```python
from build123d import *

# Parameters (mm, degrees)
SKETCH_W  = 65
SKETCH_H  = 56
SKETCH_R  = 1.35
PAD_DEPTH = 2.5
FILLET_R  = 2


with BuildPart() as part:
    # Sketch → Pad (new body)
    with BuildSketch(Plane.XY):
        Rectangle(SKETCH_W, SKETCH_H)
        with Locations((15, 15)):
            Circle(SKETCH_R, mode=Mode.SUBTRACT)
        with Locations((15, -15)):
            Circle(SKETCH_R, mode=Mode.SUBTRACT)
        with Locations((-15, -15)):
            Circle(SKETCH_R, mode=Mode.SUBTRACT)
        with Locations((-15, 15)):
            Circle(SKETCH_R, mode=Mode.SUBTRACT)
        with Locations((-29, 24.5)):
            Circle(SKETCH_R, mode=Mode.SUBTRACT)
        with Locations((29, 24.5)):
            Circle(SKETCH_R, mode=Mode.SUBTRACT)
        with Locations((29, -24.5)):
            Circle(SKETCH_R, mode=Mode.SUBTRACT)
        with Locations((-29, -24.5)):
            Circle(SKETCH_R, mode=Mode.SUBTRACT)
    extrude(amount=PAD_DEPTH)

    # Fillet
    fillet_edges = [part.edges().sort_by_distance(p)[0] for p in [
        (-32.5, -28, 1.25),
        (-32.5, 28, 1.25),
        (32.5, -28, 1.25),
        (32.5, 28, 1.25),
    ]]
    fillet(fillet_edges, radius=FILLET_R)


solid = part.part
```
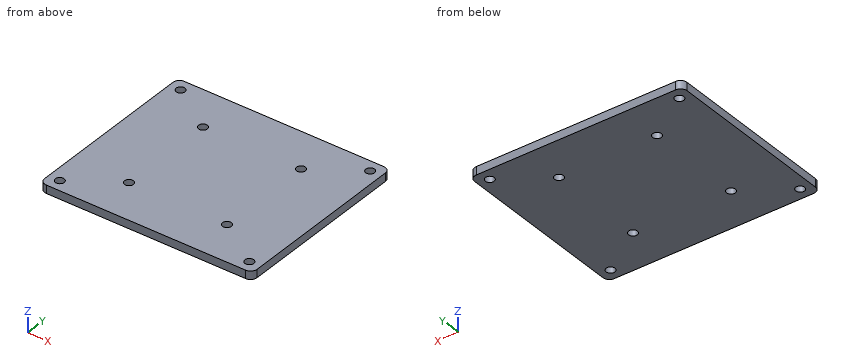
Verification items for the finished model (mm, model axes). Round coordinates to 2 decimals unless told otherwise and drop trailing zeros. Order: outer loops, then holes, each group sorted by start corner. A loop starts at its lowest first (then second) coordinate and runs counter-clockwise, first axis right, second up.
1) Cross-section at B-B, the plane y = 15. Record the cut outline in (x, z).
Geometry says:
outline: (-32.5, 0) - (-16.35, 0) - (-16.35, 2.5) - (-32.5, 2.5) - close; (-13.65, 0) - (13.65, 0) - (13.65, 2.5) - (-13.65, 2.5) - close; (16.35, 0) - (32.5, 0) - (32.5, 2.5) - (16.35, 2.5) - close
2) Cross-section at A-A, the plane x = -15. Record the cut outline in (y, z).
Geometry says:
outline: (-28, 0) - (-16.35, 0) - (-16.35, 2.5) - (-28, 2.5) - close; (-13.65, 0) - (13.65, 0) - (13.65, 2.5) - (-13.65, 2.5) - close; (16.35, 0) - (28, 0) - (28, 2.5) - (16.35, 2.5) - close
3) Material ranges on line 1 (Y direction, x = -29, z = 1.9); line 2 (Y direction, x = 15, z = 0.95); line 3 (X direction, y = -25, z = 0.5), recorded low to high.
Geometry says:
line 1: y = -28 to -25.85, -23.15 to 23.15, 25.85 to 28
line 2: y = -28 to -16.35, -13.65 to 13.65, 16.35 to 28
line 3: x = -32.5 to -30.25, -27.75 to 27.75, 30.25 to 32.5
